Can you work these out from the drawing? Everything is in mm from the part's minimum corner. A direction names the side the tool comes from. Round coordinates to 2 decimals unless told otherwise and drop trailing zeros. Loops run counter-clockwise (first coordinate to the right, second up) from the corner with the lowest first, then second, coordinate; pieces in that order, holes last. Notation, with made-up numbers: (45, 32.5) - (68, 32.5) arc R19 cw to (68, 36.5) - close; hole circle Ø1 at (-9.75, -18). An arc over 180 degrees is marked (long way). Answer as a JSON object with one key per item and string values. Group by question number.
1) If we mould it in two halves opening along Y, with no side actions, what happens to the marked faces 4, 5, 6 and 7? For each: pulls with the +Y half, pulls with the -Y half, needs draft (parallel to the pull), parting line crosses it, or undercut.
2) If I drill on line 1 along Y through (x, z) = (50, 6); line 2 along X through (y, z) = (13, 41); line 3 along Z through (x, y) = (10, 3), over which ranges is the centre line in solid material (lowest first)? Write a range as [from, to].
3) I want a section at B-B, the plane z = 13. Please give me the cut outline in (x, y), then the cut area to 3 significant figures.
4) Which directions (+Z, -Z, +X, -X, +Y, -Y) give clear straight access to the entire face, cutting with the end or side of a thin tool? Please do the marked faces 1, 2 and 3.
5) I want a section at D-D, the plane y = 70. Please give me the cut outline in (x, z), then the cut area to 3 significant figures.
6) I want a section at A-A, the plane y = 90. Please give me the cut outline in (x, z).
7) Will these pins go through, and if not, where does the flat tip stop? P1, Ø16, axis at x = 45, z = 37.5, coming from the +Y side; P2, Ø5.5, axis at x = 8.5, z = 43, coming from the +Y side; P3, Ø12, axis at x = 49, y = 89.5, coming from the +Z side.
8) I want a section at C-C, the plane x = 30. Please give me the cut outline in (y, z).
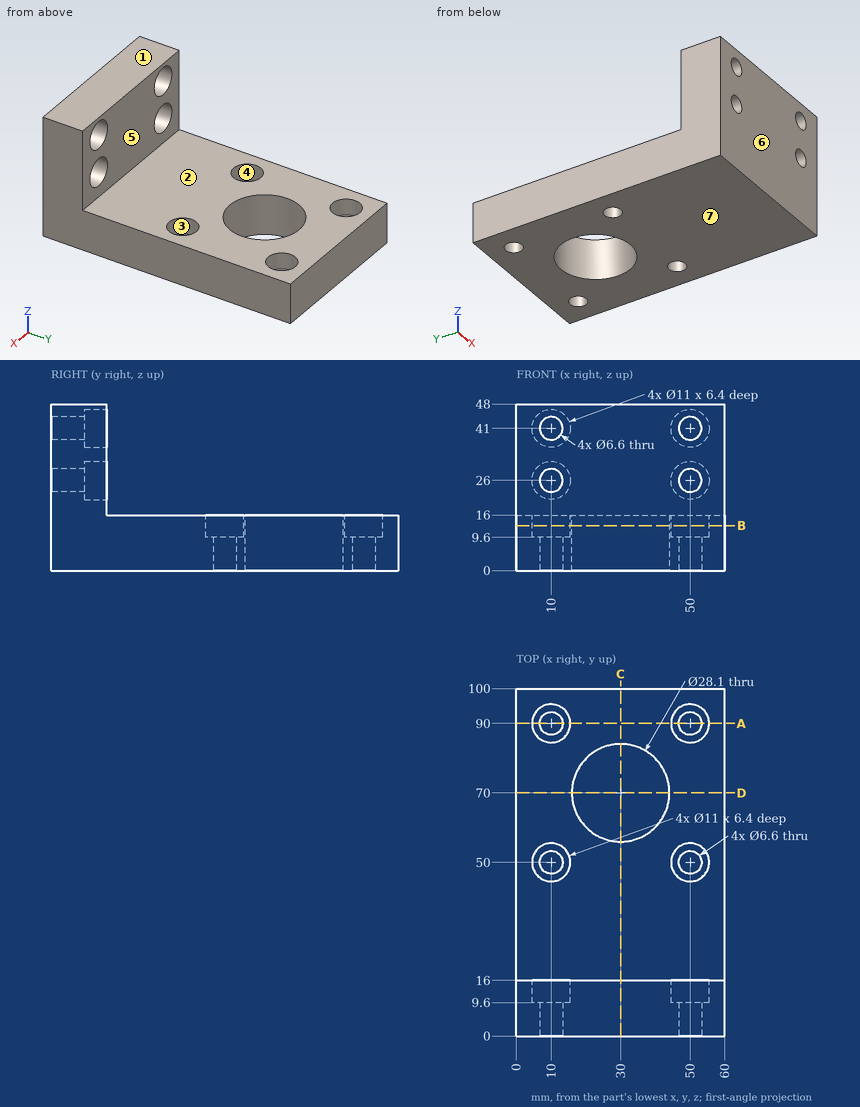
Outcome:
{
 "1": {"face 4": "undercut", "face 5": "pulls with the +Y half", "face 6": "pulls with the -Y half", "face 7": "needs draft"},
 "2": {"line 1": "[0, 46.7], [53.3, 86.7], [93.3, 100]", "line 2": "[0, 4.5], [15.5, 44.5], [55.5, 60]", "line 3": "[0, 22.7], [29.3, 37.7], [44.3, 48]"},
 "3": {"outline": "(0, 0) - (60, 0) - (60, 100) - (0, 100) - close; hole circle Ø11 at (10, 50); hole circle Ø11 at (10, 90); hole circle Ø28.1 at (30, 70); hole circle Ø11 at (50, 50); hole circle Ø11 at (50, 90)", "area": "5,000 mm^2"},
 "4": {"face 1": "+Z, +X, -X, +Y, -Y", "face 2": "+Z, +X, -X, +Y", "face 3": "+Z"},
 "5": {"outline": "(0, 0) - (15.95, 0) - (15.95, 16) - (0, 16) - close; (44.05, 0) - (60, 0) - (60, 16) - (44.05, 16) - close", "area": "510 mm^2"},
 "6": {"outline": "(0, 0) - (6.7, 0) - (6.7, 9.6) - (4.5, 9.6) - (4.5, 16) - (0, 16) - close; (13.3, 0) - (46.7, 0) - (46.7, 9.6) - (44.5, 9.6) - (44.5, 16) - (15.5, 16) - (15.5, 9.6) - (13.3, 9.6) - close; (53.3, 0) - (60, 0) - (60, 16) - (55.5, 16) - (55.5, 9.6) - (53.3, 9.6) - close"},
 "7": {"P1": "y = 16", "P2": "y = 9.6", "P3": "z = 16"},
 "8": {"outline": "(0, 0) - (55.95, 0) - (55.95, 16) - (16, 16) - (16, 48) - (0, 48) - close; (84.05, 0) - (100, 0) - (100, 16) - (84.05, 16) - close"}
}
